Geometry: final body of the model. Coordinates: model frame, mm. Give positions to 0.01 mm unless a question says otherwise; leave off trailing zeros. Write each loop counter-clockwise with the first axis right and the second up, starting at its lowest first coordinate (ties: lowest second). Pieces come first, ordered by that corner, then holes. Notation, with made-up numbers: M 41.5,30.25 L 87.5,30.25 A27 ccw 87.5,55.25 Z; hole C 80,48.5 d8. An arc over 180 degrees is marked long. Answer as a JSON object with one key per item and string values.
from build123d import *

# Parameters (mm, degrees)
BOSS_EXTRUDE1_DEPTH = 25
CUT_EXTRUDE2_DEPTH  = 55.786493398
BOSS_EXTRUDE2_DEPTH = 0.4


with BuildPart() as part:
    # Sketch1 → Boss-Extrude1 (new body)
    with BuildSketch(Plane(origin=(0, 0, 0), x_dir=(1, 0, 0), z_dir=(0, 1, 0))):
        with BuildLine():
            ThreePointArc((1.451818925, -34.068556857), (1.641248992, -34.346908706), (1.964225605, -34.442038138))
            ThreePointArc((1.964225605, -34.442038138), (26.591847487, -21.978073076), (34.198225299, 4.555174015))
            ThreePointArc((34.198225299, 4.555174015), (23.590291339, 25.176355888), (2.324135821, 34.423627607))
            ThreePointArc((2.324135821, 34.423627607), (1.751838249, 34.289058819), (1.354061739, 33.856153382))
            ThreePointArc((1.354061739, 33.856153382), (0, 33.001534515), (-1.354061739, 33.856153382))
            ThreePointArc((-1.354061739, 33.856153382), (-1.751838249, 34.289058819), (-2.324135821, 34.423627607))
            ThreePointArc((-2.324135821, 34.423627607), (-23.590291339, 25.176355888), (-34.198225299, 4.555174015))
            ThreePointArc((-34.198225299, 4.555174015), (-26.591847487, -21.978073076), (-1.964225605, -34.442038138))
            ThreePointArc((-1.964225605, -34.442038138), (-1.641248992, -34.346908706), (-1.451818925, -34.068556857))
            ThreePointArc((-1.451818925, -34.068556857), (0, -32.945679925), (1.451818925, -34.068556857))
        make_face()
        with BuildLine():
            Line((-2.417, 3.787737139), (0, 3.787737139))
            Line((0, 3.787737139), (2.417, 3.787737139))
            ThreePointArc((2.417, 3.787737139), (0, -4.489512172), (-2.417, 3.787737139))
        make_face(mode=Mode.SUBTRACT)
    extrude(amount=BOSS_EXTRUDE1_DEPTH)

    # Sketch2 → Cut-Extrude2 (cut, through all)
    with BuildSketch(Plane(origin=(0, 0, 0), x_dir=(1, 0, 0), z_dir=(0, 1, 0))):
        with BuildLine():
            ThreePointArc((-31.8625, -2.963291034), (-22.627416998, -22.627416998), (-2.963291034, -31.8625))
            ThreePointArc((-2.963291034, -31.8625), (-1.977020771, -31.703659042), (-1.190608005, -31.087611607))
            ThreePointArc((-1.190608005, -31.087611607), (0, -30.5), (1.190608005, -31.087611607))
            ThreePointArc((1.190608005, -31.087611607), (1.977020771, -31.703659042), (2.963291034, -31.8625))
            ThreePointArc((2.963291034, -31.8625), (22.627416998, -22.627416998), (31.8625, -2.963291034))
            ThreePointArc((31.8625, -2.963291034), (31.703659042, -1.977020771), (31.087611607, -1.190608005))
            ThreePointArc((31.087611607, -1.190608005), (30.5, 0), (31.087611607, 1.190608005))
            ThreePointArc((31.087611607, 1.190608005), (31.703659042, 1.977020771), (31.8625, 2.963291034))
            ThreePointArc((31.8625, 2.963291034), (22.627416998, 22.627416998), (2.963291034, 31.8625))
            ThreePointArc((2.963291034, 31.8625), (1.977020771, 31.703659042), (1.190608005, 31.087611607))
            ThreePointArc((1.190608005, 31.087611607), (0, 30.5), (-1.190608005, 31.087611607))
            ThreePointArc((-1.190608005, 31.087611607), (-1.977020771, 31.703659042), (-2.963291034, 31.8625))
            ThreePointArc((-2.963291034, 31.8625), (-22.627416998, 22.627416998), (-31.8625, 2.963291034))
            ThreePointArc((-31.8625, 2.963291034), (-31.703659042, 1.977020771), (-31.087611607, 1.190608005))
            ThreePointArc((-31.087611607, 1.190608005), (-30.5, 0), (-31.087611607, -1.190608005))
            ThreePointArc((-31.087611607, -1.190608005), (-31.703659042, -1.977020771), (-31.8625, -2.963291034))
        make_face()
    extrude(amount=CUT_EXTRUDE2_DEPTH, mode=Mode.SUBTRACT)

    # Sketch2<2> → Boss-Extrude2 (add)
    with BuildSketch(Plane(origin=(0, 0, 0), x_dir=(1, 0, 0), z_dir=(0, 1, 0))):
        with BuildLine():
            ThreePointArc((-31.8625, -2.963291034), (-22.627416998, -22.627416998), (-2.963291034, -31.8625))
            ThreePointArc((-2.963291034, -31.8625), (-1.977020771, -31.703659042), (-1.190608005, -31.087611607))
            ThreePointArc((-1.190608005, -31.087611607), (0, -30.5), (1.190608005, -31.087611607))
            ThreePointArc((1.190608005, -31.087611607), (1.977020771, -31.703659042), (2.963291034, -31.8625))
            ThreePointArc((2.963291034, -31.8625), (22.627416998, -22.627416998), (31.8625, -2.963291034))
            ThreePointArc((31.8625, -2.963291034), (31.703659042, -1.977020771), (31.087611607, -1.190608005))
            ThreePointArc((31.087611607, -1.190608005), (30.5, 0), (31.087611607, 1.190608005))
            ThreePointArc((31.087611607, 1.190608005), (31.703659042, 1.977020771), (31.8625, 2.963291034))
            ThreePointArc((31.8625, 2.963291034), (22.627416998, 22.627416998), (2.963291034, 31.8625))
            ThreePointArc((2.963291034, 31.8625), (1.977020771, 31.703659042), (1.190608005, 31.087611607))
            ThreePointArc((1.190608005, 31.087611607), (0, 30.5), (-1.190608005, 31.087611607))
            ThreePointArc((-1.190608005, 31.087611607), (-1.977020771, 31.703659042), (-2.963291034, 31.8625))
            ThreePointArc((-2.963291034, 31.8625), (-22.627416998, 22.627416998), (-31.8625, 2.963291034))
            ThreePointArc((-31.8625, 2.963291034), (-31.703659042, 1.977020771), (-31.087611607, 1.190608005))
            ThreePointArc((-31.087611607, 1.190608005), (-30.5, 0), (-31.087611607, -1.190608005))
            ThreePointArc((-31.087611607, -1.190608005), (-31.703659042, -1.977020771), (-31.8625, -2.963291034))
        make_face()
    extrude(amount=BOSS_EXTRUDE2_DEPTH)


solid = part.part
1) Contact query for flat-ended pins moving along their axis: P1, Ø6, axis at x = 20.5, y = 5.5, coming from the -Z side; P2, Ø4, axis at x = -14, z = -11.5, coming from the +Y side; P3, Ø1, axis at y = 7.5, z = 4.5, coming from the +X side. Output: stop coordinate, or through.
Geometry check:
{"P1": "stops at z = -29.73", "P2": "stops at y = 0.4", "P3": "stops at x = 34.27"}
2) Pull-direction query (Z, two-part tool) for faces 1 (the flat face through (0, 0.4, 0)), 2 (the cylindrical face through (-0.028, 12.325, 32.946)), 3 (the flat face through (-31, 25, 0)), 4 (the cylindrical face through (0, 12, -33)); classes: pulls with the +Z half, pulls with the -Z half, needs draft (parallel to the pull), parting line crosses it, or undercut.
Geometry check:
{"face 1": "undercut", "face 2": "pulls with the +Z half", "face 3": "needs draft", "face 4": "pulls with the -Z half"}
3) Line query: line 1 (Y direction, x = 6.5, z = 1.5); line 2 (X direction, y = 11.5, z = -2); line 3 (X direction, y = 12.5, z = 6). Output: solid intervals per line, ascending. Write a range as from..to.
Geometry check:
{"line 1": "y = 0..0.4", "line 2": "x = -34.44..-31.71, 31.71..34.44", "line 3": "x = -33.97..-31.43, 31.43..33.97"}
4) Cut plane B-B on z = 23. Return loops of the section in (x, y).
Geometry check:
{"outline": "M -25.71,0 L 25.71,0 L 25.71,25 L 22.25,25 L 22.25,0.4 L -22.25,0.4 L -22.25,25 L -25.71,25 Z"}
5) Cut plane C-C on x = 5. Return loops of the section in (y, z).
Geometry check:
{"outline": "M 0,-34.14 L 25,-34.14 L 25,-31.61 L 0.4,-31.61 L 0.4,31.61 L 25,31.61 L 25,34.13 L 0,34.13 Z"}
